Input: part model. Units: mm. Frame: model coordinates. A direction names the side the tool comes from. Round coordinates to 2 decimals unless told otherwise and drop trailing zeros. Loops run counter-clockwise (first coordinate to the right, second up) from the corner with the lowest first, then second, coordinate; pieces in that order, holes last. Notation, with made-up numbers: M -25.5,-23.5 L 29.5,-23.5 A24 cw 29.5,12.5 Z; hole C 37,76 d7. An arc over 180 degrees is marked long. Use one line per item in the form item = value. Start each with the question number.
Q1. Access query for faces 5 (the flat face through (9, 27, 2.55)), 6 (the flat face through (-1, 27, 2.55)), 7 (the flat face through (4, 13, 7)). Directions: +Z, -Z, +X, -X, +Y, -Y. A direction counts if a zero-diameter tool reaches every point of the face in a straight line with its end or side. Return the directions, or none.
Q2. Section query D-D, the plane x = -1.25. Output: boundary loops of the cut face in (y, z), and give its area (3 significant figures).
Q3. Mould query, pull axis X, two halves, no side actions, for faces 1 (the flat face through (7.92, 27, 2)), 2 (the cylindrical face through (3.85, 6.92, 4.85)), 3 (the flat face through (0, 27, 2)), 4 (the flat face through (3.9, 0.5, 8.469)). Classes: pulls with the +X half, pulls with the -X half, needs draft (parallel to the pull), parting line crosses it, or undercut.
Q4. Ray query, line 1 along Y through (x, z) = (2, 5.5); line 2 along Y through (x, z) = (9, 7); line 3 along Y through (x, z) = (7.5, 1.5). Return the intervals inside material, ascending.
Q5. Section query A-A, the plane y = 42.5. Output: boundary loops of the cut face in (x, z), and give its area (3 significant figures).
Q6. Section query B-B, the plane x = 3.96. Output: boundary loops of the cut face in (y, z) (3 decimals).
Q7. First-contact query: P1, Ø1.8, axis at x = 3.5, y = -1.5, coming from the -Z side; P2, Ø1.7, axis at y = 26.5, z = 1.5, coming from the -X side; P3, Ø1.5, axis at x = 2.5, y = 9, coming from the +Z side. Flat tips, straight axial feed; report the tip coordinate or a pass-through.
Q8. Section query C-C, the plane x = 10. Output: boundary loops of the cut face in (y, z), and give its area (3 significant figures).
```python
from build123d import *

# Parameters (mm, degrees)
BOSS_EXTRUDE1_DEPTH = 54.32
FILLET1_R           = 1
BOSS_EXTRUDE2_DEPTH = 5
SKETCH3_R           = 8.5
CUT_EXTRUDE1_DEPTH  = 13
BOSS_EXTRUDE3_DEPTH = 1


with BuildPart() as part:
    # Sketch1 → Boss-Extrude1 (new body)
    with BuildSketch(Plane(origin=(0, 0, 0), x_dir=(1, 0, 0), z_dir=(0, 1, 0))):
        Polygon((10.92, -2.55), (7.92, -2.55), (7.92, 0), (0, 0), (0, -2.55), (-3, -2.55), (-3, -8.55), (10.92, -8.55), align=None)
    extrude(amount=BOSS_EXTRUDE1_DEPTH)

    # Fillet1
    fillet1_edges = [part.edges().sort_by_distance(p)[0] for p in [
        (0, 27.16, 0),
        (7.92, 27.16, 0),
    ]]
    fillet(fillet1_edges, radius=FILLET1_R)

    # Sketch2 → Boss-Extrude2 (add)
    with BuildSketch(Plane(origin=(0, 54.32, 0), x_dir=(1, 0, 0), z_dir=(0, 1, 0))):
        with BuildLine():
            Line((5.736407892, -2.05), (2.183592108, -2.05))
            ThreePointArc((2.183592108, -2.05), (2.863703077, -6.490032388), (6.635, -4.05))
            ThreePointArc((6.635, -4.05), (6.400032388, -2.953703077), (5.736407892, -2.05))
        make_face()
    boss_extrude2 = extrude(amount=BOSS_EXTRUDE2_DEPTH)

    # Mirror1: Boss-Extrude2 across plane
    add(boss_extrude2.mirror(Plane.ZX.offset(27.16)))

    # Sketch3 → Cut-Extrude1 (cut)
    with BuildSketch(Plane.XZ):
        with Locations((3.96, 13.348484692)):
            Circle(SKETCH3_R)
    extrude(amount=-CUT_EXTRUDE1_DEPTH, mode=Mode.SUBTRACT)

    # Sketch4 → Boss-Extrude3 (add)
    with BuildSketch(Plane(origin=(0, 0, 0), x_dir=(1, 0, 0), z_dir=(0, 1, 0))):
        with BuildLine():
            Line((-3, -8.469099485), (10.92, -8.469099485))
            ThreePointArc((10.92, -8.469099485), (8.9248008, -6.449154796), (6.375674383, -5.198974445))
            ThreePointArc((6.375674383, -5.198974445), (3.96, -4.848484692), (1.544325617, -5.198974445))
            ThreePointArc((1.544325617, -5.198974445), (-1.0048008, -6.449154796), (-3, -8.469099485))
        make_face()
    extrude(amount=BOSS_EXTRUDE3_DEPTH)


solid = part.part
```
Results found:
q1.face_5 = -Z, +X, +Y, -Y
q1.face_6 = -Z, -X, +Y, -Y
q1.face_7 = +Z
q2.outline = M 0,2.55 L 54.32,2.55 L 54.32,8.55 L 13,8.55 L 13,6.63 L 1,6.63 L 1,8.47 L 0,8.47 Z
q2.area = 303 mm²
q3.face_1 = pulls with the +X half
q3.face_2 = undercut
q3.face_3 = pulls with the -X half
q3.face_4 = needs draft
q4.line_1 = -5 to 1, 13 to 59.32
q4.line_2 = 0 to 1, 13 to 54.32
q4.line_3 = 0 to 54.32
q5.outline = M -3,2.55 L 0,2.55 L 0,1 A1 ccw 1,0 L 6.92,0 A1 ccw 7.92,1 L 7.92,2.55 L 10.92,2.55 L 10.92,8.55 L -3,8.55 Z
q5.area = 103 mm²
q6.outline = M -5,2.05 L 0,2.05 L 0,0 L 54.32,0 L 54.32,2.05 L 59.32,2.05 L 59.32,6.725 L 54.32,6.725 L 54.32,8.55 L 13,8.55 L 13,4.848 L 1,4.848 L 1,8.469 L 0,8.469 L 0,6.725 L -5,6.725 Z
q7.P1 = 2.05
q7.P2 = 0
q7.P3 = 5.14
q8.outline = M 0,2.55 L 54.32,2.55 L 54.32,8.55 L 13,8.55 L 13,7.37 L 1,7.37 L 1,8.47 L 0,8.47 Z
q8.area = 312 mm²
